Input: dimensioned drawing with shaded views. Units: mm. Origin: part minimum x, y, z. A direction names the side the tool comes from. Coordinates: 2 decimals unless noted, no trailing zeros. Write each loop counter-clockwise with the first axis right and the second up, starting at its lowest first coordinate (ties: lowest second). Pieces come first, ordered by that corner, then holes. Notation, with made-up numbers: M 27,-23 L 86,-23 A22 cw 86,1 Z; hole C 63,22 d10. An arc over 180 degrees is marked long. Use one line per item in the form item = value.
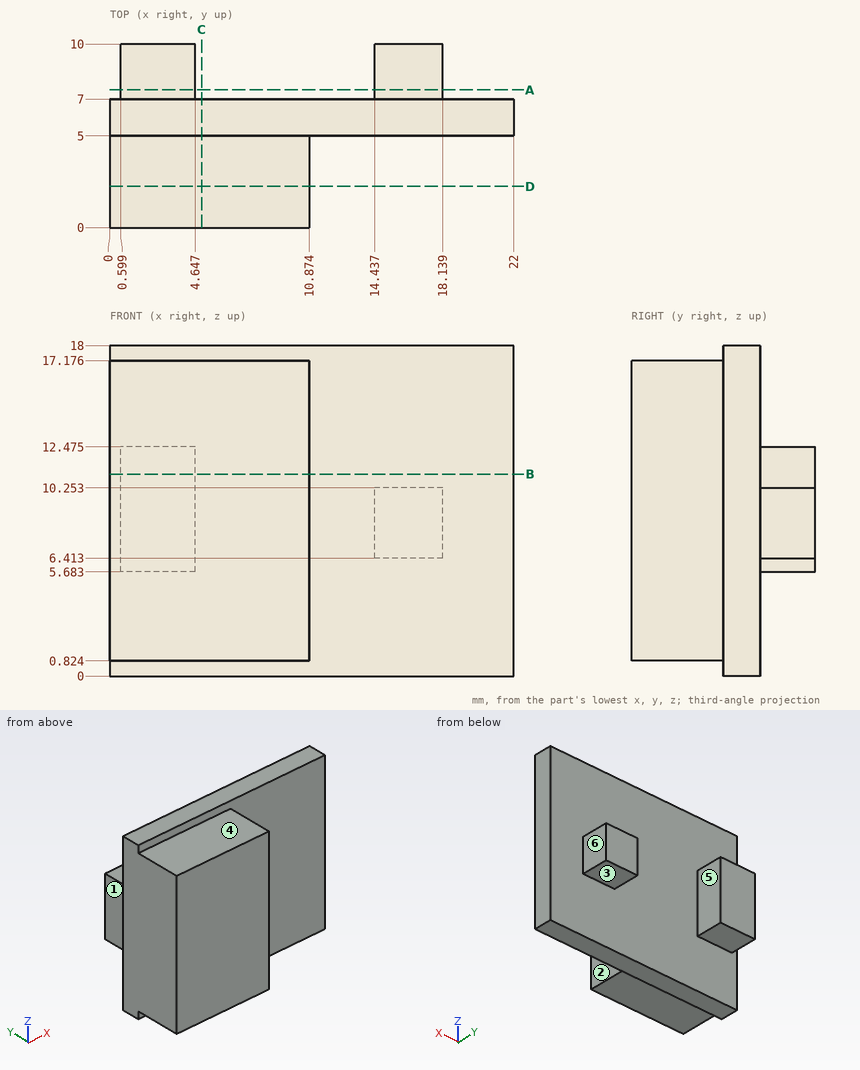
(1) Section query C-C on x = 5. Return the cut outline in (y, z) (1 decimal).
Computed:
outline = M 0,0.8 L 5,0.8 L 5,0 L 7,0 L 7,18 L 5,18 L 5,17.2 L 0,17.2 Z
(2) Set-up query: the marked faces 1, 2 and 3. Return all of +Z, -Z, +X, -X, +Y, -Y with unobstructed straight access to the full face (end or side cutting, diameter ignored); none if empty.
Computed:
face_1 = +Z, -Z, -X, +Y
face_2 = +Z, -Z, +X, -Y
face_3 = -Z, +X, +Y
(3) Line query: probe 1 along X at (y, z) = (8.75, 7); probe 2 along Y at (x, z) = (5.5, 6); probe 3 along Y at (x, z) = (12.5, 2.5). Output: solid intervals per line, ascending.
Computed:
probe_1 = 0.6 to 4.65, 14.44 to 18.14
probe_2 = 0 to 7
probe_3 = 5 to 7
(4) Pull-direction query (X, two-part tool) for the marked faces 4, 5 and 6; classes: pulls with the +X half, pulls with the -X half, needs draft (parallel to the pull), parting line crosses it, or undercut.
Computed:
face_4 = needs draft
face_5 = undercut
face_6 = pulls with the +X half
(5) Section query B-B on z = 11. Return the cut outline in (x, y) (1 decimal).
Computed:
outline = M 0,0 L 10.9,0 L 10.9,5 L 22,5 L 22,7 L 4.6,7 L 4.6,10 L 0.6,10 L 0.6,7 L 0,7 Z
(6) Section query A-A on y = 7.5. Return the cut outline in (x, z) (1 decimal).
Computed:
outline = M 0.6,5.7 L 4.6,5.7 L 4.6,12.5 L 0.6,12.5 Z; M 14.4,6.4 L 18.1,6.4 L 18.1,10.3 L 14.4,10.3 Z
(7) Section query D-D on y = 2.25. Return the cut outline in (x, z) (1 decimal).
Computed:
outline = M 0,0.8 L 10.9,0.8 L 10.9,17.2 L 0,17.2 Z
(8) First-contact query: pin 1 Ø0.9 at (y, z) = (9, 7.5) entering from -X; pin 2 Ø0.9 at (x, y) = (16, 8) entering from +Z; pin 3 Ø1.5 at (y, z) = (8, 7) entering from +X. Flat tips, straight axial feed; report the tip coordinate or a pass-through.
Computed:
pin_1 = 0.6
pin_2 = 10.25
pin_3 = 18.14
